CAD build for the part. Positions are in the model's coordinates, mm. A direction names the side the tool comes from. Coordinates: 2 decimals unless noted, no trailing zeros. Order: outer loops, then holes, each group sorted by start corner. A loop starts at its lowest first (then second) coordinate and runs counter-clockwise, first axis right, second up. Notation, with made-up numbers: M 41.5,-4.5 L 55.5,-4.5 A24 cw 55.5,13.5 Z; hole C -13.75,52.5 d11. An arc over 180 degrees is marked long. One line per item, written item: value.
from build123d import *

# Parameters (mm, degrees)
SKETCH1_R           = 7
BOSS_EXTRUDE1_DEPTH = 12
SKETCH2_R           = 2.55
CUT_EXTRUDE1_DEPTH  = 1
SKETCH3_R           = 1.5
CUT_EXTRUDE2_DEPTH  = 4
CUT_EXTRUDE3_DEPTH  = 2
SKETCH5_W           = 6.350852962
SKETCH5_H           = 2
CUT_EXTRUDE4_DEPTH  = 5
SKETCH5_2_W         = 6.350852962
SKETCH5_2_H         = 2
CUT_EXTRUDE5_DEPTH  = 2.7
SKETCH6_R           = 1.5
CUT_EXTRUDE6_DEPTH  = 7
BOSS_EXTRUDE2_DEPTH = 12
CUT_EXTRUDE7_DEPTH  = 12
CUT_EXTRUDE8_DEPTH  = 12


with BuildPart() as part:
    # Sketch1 → Boss-Extrude1 (new body)
    with BuildSketch(Plane.XY):
        Circle(SKETCH1_R)
    extrude(amount=BOSS_EXTRUDE1_DEPTH)

    # Sketch2 → Cut-Extrude1 (cut)
    with BuildSketch(Plane.XY.offset(12)):
        Circle(SKETCH2_R)
    extrude(amount=-CUT_EXTRUDE1_DEPTH, mode=Mode.SUBTRACT)

    # Sketch3 → Cut-Extrude2 (cut)
    with BuildSketch(Plane(origin=(0, 0, 0), x_dir=(-1, 0, 0), z_dir=(0, 0, -1))):
        Circle(SKETCH3_R)
    extrude(amount=-CUT_EXTRUDE2_DEPTH, mode=Mode.SUBTRACT)

    # Sketch4 → Cut-Extrude3 (cut)
    with BuildSketch(Plane(origin=(0, 0, 4), x_dir=(-1, 0, 0), z_dir=(0, 0, -1))):
        Polygon((0, 3.175426481), (-2.75, 1.58771324), (-2.75, -1.58771324), (0, -3.175426481), (2.75, -1.58771324), (2.75, 1.58771324), align=None)
    extrude(amount=CUT_EXTRUDE3_DEPTH, mode=Mode.SUBTRACT)

    # Sketch5 → Cut-Extrude4 (cut)
    with BuildSketch(Plane(origin=(-1.375, 2.38156986, 0), x_dir=(0.866025404, 0.5, 0), z_dir=(0.5, -0.866025404, 0))):
        with Locations((0, 3)):
            Rectangle(SKETCH5_W, SKETCH5_H)
    extrude(amount=-CUT_EXTRUDE4_DEPTH, mode=Mode.SUBTRACT)

    # Sketch5<2> → Cut-Extrude5 (cut)
    with BuildSketch(Plane(origin=(-1.375, 2.38156986, 0), x_dir=(0.866025404, 0.5, 0), z_dir=(0.5, -0.866025404, 0))):
        with Locations((0, 3)):
            Rectangle(SKETCH5_2_W, SKETCH5_2_H)
    extrude(amount=CUT_EXTRUDE5_DEPTH, mode=Mode.SUBTRACT)

    # Sketch6 → Cut-Extrude6 (cut)
    with BuildSketch(Plane(origin=(0, 0, 0), x_dir=(-1, 0, 0), z_dir=(0, 0, -1))):
        Circle(SKETCH6_R)
    extrude(amount=-CUT_EXTRUDE6_DEPTH, mode=Mode.SUBTRACT)

    # Sketch7 → Boss-Extrude2 (add)
    with BuildSketch(Plane.XY.offset(12)):
        with BuildLine():
            Line((-5.869161212, 3.814832456), (-6.25, 4.474464586))
            Line((-6.25, 4.474464586), (-7, 4.041451884))
            Line((-7, 4.041451884), (-7, 0))
            ThreePointArc((-7, 0), (-6.711338484, 1.989456146), (-5.869161212, 3.814832456))
        make_face()
        with BuildLine():
            Line((3.499999838, 6.06217792), (0, 8.082903769))
            Line((0, 8.082903769), (-0.75, 7.649891067))
            Line((-0.75, 7.649891067), (-0.369161212, 6.990258937))
            ThreePointArc((-0.369161212, 6.990258937), (1.632749589, 6.806917715), (3.499999838, 6.06217792))
        make_face()
        with BuildLine():
            Line((7, 4.041451884), (3.499999838, 6.06217792))
            ThreePointArc((3.499999838, 6.06217792), (6.06217778, 3.500000081), (7, 0))
            Line((7, 0), (7, 4.041451884))
        make_face()
        with BuildLine():
            Line((7, -4.041451884), (7, 0))
            ThreePointArc((7, 0), (6.062177778, -3.500000084), (3.499999831, -6.062177924))
            Line((3.499999831, -6.062177924), (7, -4.041451884))
        make_face()
        with BuildLine():
            Line((0, -8.082903769), (3.499999831, -6.062177924))
            ThreePointArc((3.499999831, -6.062177924), (-1.13e-07, -7), (-3.500000026, -6.062177811))
            Line((-3.500000026, -6.062177811), (0, -8.082903769))
        make_face()
        with BuildLine():
            ThreePointArc((-3.500000026, -6.062177811), (-6.062177834, -3.499999987), (-7, 0))
            Line((-7, 0), (-7, -4.041451884))
            Line((-7, -4.041451884), (-3.500000026, -6.062177811))
        make_face()
    extrude(amount=-BOSS_EXTRUDE2_DEPTH)

    # Sketch7<4> → Cut-Extrude7 (cut)
    with BuildSketch(Plane.XY.offset(12)):
        with BuildLine():
            ThreePointArc((-0.369161212, 6.990258937), (-1.989456099, 6.711338498), (-3.499999915, 6.062177876))
            ThreePointArc((-3.499999915, 6.062177876), (-4.817461512, 5.078588838), (-5.869161212, 3.814832456))
            Line((-5.869161212, 3.814832456), (-0.369161212, 6.990258937))
        make_face()
    extrude(amount=-CUT_EXTRUDE7_DEPTH, mode=Mode.SUBTRACT)

    # Sketch8 → Cut-Extrude8 (cut)
    with BuildSketch(Plane.XY.offset(12)):
        Polygon((-7, 3.161942377), (-5.869161212, 3.814832456), (-6.25, 4.474464586), (-7, 4.041451884), align=None)
        Polygon((-0.75, 7.649891067), (-0.369161212, 6.990258937), (0.761677576, 7.643149015), (0, 8.082903769), align=None)
    extrude(amount=-CUT_EXTRUDE8_DEPTH, mode=Mode.SUBTRACT)


solid = part.part
Q1. Slice it at A-A (z = 1.75). List the corners of the cut face in (x, y), plus the area to 3 significant figures.
Recorded:
outline: M -7,-4.04 L 0,-8.08 L 7,-4.04 L 7,4.04 L 0.76,7.64 L -7,3.16 Z; hole C 0,0 d3
area: 156 mm^2
Q2. Slice it at B-B (z = 9). List the corners of the cut face in (x, y).
Recorded:
outline: M -7,-4.04 L 0,-8.08 L 7,-4.04 L 7,4.04 L 0.76,7.64 L -7,3.16 Z
Q3. Slice it at C-C (x = -4.25). List the corners of the cut face in (y, z).
Recorded:
outline: M -5.63,0 L 4.75,0 L 4.75,2 L 1.01,2 L 1.01,4 L 4.75,4 L 4.75,12 L -5.63,12 Z
Q4. Pin check, flat tips, straight feed: pin 1 Ø2.5 at (x, y) = (-0.5, -0.5) entering from -Z; pin 2 Ø2.5 at (x, y) = (0, 0) entering from +Z; pin 3 Ø1.5 at (x, z) = (-3.5, 3.5) entering from -Y; pin 4 Ø2 at (x, z) = (0.5, 7) entering from -Y. Stop position of each tip, or through.
Recorded:
pin 1: stops at z = 0
pin 2: stops at z = 11
pin 3: stops at y = -6.5
pin 4: stops at y = -8.08
Q5. Mould opens along Y. For faces 6 (the face through (-4.3, 1.1, 3)), 7 (the face through (2.75, 0, 3)), 8 (the face through (1.18, -2.26, 11.51)), 9 (the face through (7, 0, 6)) say: released by +Y, released by -Y, zero draft, split by the parting line, or undercut.
Recorded:
face 6: released by +Y
face 7: undercut
face 8: undercut
face 9: zero draft
Q6. Which spindle directions (+Z, -Z, +X, -X, +Y, -Y) get a long thin tool onto all of the face, cutting with end or side? Do faces 1 (the face through (-7, 0, 6)), 2 (the face through (1.5, 0.07, 0.99)), 3 (the face through (-1, 2, 2)), 4 (the face through (0, -2, 0)), 5 (the face through (0, 0, 11)). Say none if no direction does.
Recorded:
face 1: +Z, -Z, -X, +Y, -Y
face 2: -Z
face 3: none
face 4: -Z, +X, -X, +Y, -Y
face 5: +Z
Q7. Slice it at D-D (y = 0). List the corners of the cut face in (x, z).
Recorded:
outline: M -7,0 L -1.5,0 L -1.5,2 L -3.67,2 L -3.67,4 L -1.5,4 L -1.5,7 L 1.5,7 L 1.5,4 L 2.75,4 L 2.75,2 L 1.5,2 L 1.5,0 L 7,0 L 7,12 L 2.55,12 L 2.55,11 L -2.55,11 L -2.55,12 L -7,12 Z
Q8. Drill centre lines: line 1 along Y through (x, z) = (3.5, 6); line 2 along Z through (x, y) = (1, 0.5); line 3 along Y through (x, z) = (6.5, 9). Where is each one in solid material? Low to high.
Recorded:
line 1: y = -6.06 to 6.06
line 2: z = 7 to 11
line 3: y = -4.33 to 4.33
